Work out the finished part from the listing and answer in its coordinate system (mm). A direction names the side the tool comes from. Round coordinates to 2 decimals unless told otherwise and drop trailing zeros. Write each loop counter-clockwise with the first axis right and the second up, starting at its lowest first coordinate (ties: lowest second). Pieces come first, ordered by that corner, then holes.
from build123d import *

# Parameters (mm, degrees)
SKETCH1_W               = 160
SKETCH1_H               = 45
BOSS_EXTRUDE1_DEPTH     = 28
SKETCH3_W               = 65
SKETCH3_H               = 25
CUT_EXTRUDE2_DEPTH      = 28
CUT_EXTRUDE3_DEPTH      = 28
SKETCH8_R               = 2
CUT_EXTRUDE4_DEPTH      = 10
CUT_EXTRUDE5_DEPTH      = 169.549695936
CUT_EXTRUDE5_DEPTH_BACK = 169.549695936
SKETCH9_W               = 16
SKETCH9_H               = 28
SKETCH10_W              = 128
SKETCH10_H              = 5.5
CUT_EXTRUDE6_DEPTH      = 154.443800787
SKETCH11_W              = 128
SKETCH11_H              = 2.75
CUT_EXTRUDE7_DEPTH      = 152.921854912
SKETCH12_W              = 128
SKETCH12_H              = 2.75
BOSS_EXTRUDE3_DEPTH     = 28
SKETCH13_R              = 2
CUT_EXTRUDE8_DEPTH      = 152.230163989
SKETCH14_W              = 128
SKETCH14_H              = 28
BOSS_EXTRUDE4_DEPTH     = 2
SKETCH16_R              = 2
CUT_EXTRUDE9_DEPTH      = 152.230163989


with BuildPart() as part:
    # Sketch1 → Boss-Extrude1 (new body)
    with BuildSketch(Plane.XY):
        with Locations((80, 22.5)):
            Rectangle(SKETCH1_W, SKETCH1_H)
    extrude(amount=BOSS_EXTRUDE1_DEPTH)

    # Sketch3 → Cut-Extrude2 (cut)
    with BuildSketch(Plane.XY.offset(28)):
        with Locations((32.5, 21.5)):
            Rectangle(SKETCH3_W, SKETCH3_H)
        with Locations((127.5, 21.5)):
            Rectangle(SKETCH3_W, SKETCH3_H)
    extrude(amount=-CUT_EXTRUDE2_DEPTH, mode=Mode.SUBTRACT)

    # Sketch6 → Cut-Extrude3 (cut)
    with BuildSketch(Plane.XZ):
        Polygon((65, 14), (65, 24), (25, 24), (25, 4), (65, 4), align=None)
        Polygon((95, 4), (95, 14), (95, 24), (135, 24), (135, 4), align=None)
    extrude(amount=-CUT_EXTRUDE3_DEPTH, mode=Mode.SUBTRACT)

    # Sketch8 → Cut-Extrude4 (cut)
    with BuildSketch(Plane(origin=(0, 0, 0), x_dir=(-1, 0, 0), z_dir=(0, -1, 0))):
        with Locations(Location((-20.5, -9, 0), (0, 0, 90))):
            Circle(SKETCH8_R)
        with Locations(Location((-20.5, -19, 0), (0, 0, 90))):
            Circle(SKETCH8_R)
        with Locations(Location((-90.5, -19, 0), (0, 0, 90))):
            Circle(SKETCH8_R)
        with Locations(Location((-90.5, -9, 0), (0, 0, 90))):
            Circle(SKETCH8_R)
        with Locations(Location((-139.5, -19, 0), (0, 0, 90))):
            Circle(SKETCH8_R)
        with Locations(Location((-139.5, -9, 0), (0, 0, 90))):
            Circle(SKETCH8_R)
        with Locations(Location((-69.5, -19, 0), (0, 0, 90))):
            Circle(SKETCH8_R)
        with Locations(Location((-69.5, -9, 0), (0, 0, 90))):
            Circle(SKETCH8_R)
    extrude(amount=-CUT_EXTRUDE4_DEPTH, mode=Mode.SUBTRACT)

    # Sketch9 → Cut-Extrude5 (cut, two sides: drawn at the far end of the back side and taken through both)
    with BuildSketch(Plane(origin=(0, 0, 0), x_dir=(-1, 0, 0), z_dir=(0, -1, 0)).offset(-CUT_EXTRUDE5_DEPTH_BACK)):
        with Locations((-152, -14)):
            Rectangle(SKETCH9_W, SKETCH9_H)
        with Locations((-8, -14)):
            Rectangle(SKETCH9_W, SKETCH9_H)
    extrude(amount=CUT_EXTRUDE5_DEPTH + CUT_EXTRUDE5_DEPTH_BACK, mode=Mode.SUBTRACT)

    # Sketch10 → Cut-Extrude6 (cut, through all)
    with BuildSketch(Plane.XY.offset(28)):
        with Locations((80, 42.25)):
            Rectangle(SKETCH10_W, SKETCH10_H)
    extrude(amount=-CUT_EXTRUDE6_DEPTH, mode=Mode.SUBTRACT)

    # Sketch11 → Cut-Extrude7 (cut, through all)
    with BuildSketch(Plane.XY.offset(28)):
        with Locations((80, 38.125)):
            Rectangle(SKETCH11_W, SKETCH11_H)
    extrude(amount=-CUT_EXTRUDE7_DEPTH, mode=Mode.SUBTRACT)

    # Sketch12 → Boss-Extrude3 (add)
    with BuildSketch(Plane.XY.offset(28)):
        with Locations((80, 32.625)):
            Rectangle(SKETCH12_W, SKETCH12_H)
    extrude(amount=-BOSS_EXTRUDE3_DEPTH)

    # Sketch13 → Cut-Extrude8 (cut, through all)
    with BuildSketch(Plane(origin=(0, 36.75, 0), x_dir=(1, 0, 0), z_dir=(0, 1, 0))):
        with Locations(Location((125, -14, 0), (0, 0, 270))):
            Circle(SKETCH13_R)
        with Locations(Location((35, -14, 0), (0, 0, 270))):
            Circle(SKETCH13_R)
    extrude(amount=-CUT_EXTRUDE8_DEPTH, mode=Mode.SUBTRACT)

    # Sketch14 → Boss-Extrude4 (add)
    with BuildSketch(Plane(origin=(0, 36.75, 0), x_dir=(1, 0, 0), z_dir=(0, 1, 0))):
        with Locations((80, -14)):
            Rectangle(SKETCH14_W, SKETCH14_H)
    extrude(amount=BOSS_EXTRUDE4_DEPTH)

    # Sketch16 → Cut-Extrude9 (cut, through all)
    with BuildSketch(Plane.XZ.offset(-36.75)):
        with Locations(Location((125, 14, 0), (0, 0, 90))):
            Circle(SKETCH16_R)
        with Locations(Location((35, 14, 0), (0, 0, 90))):
            Circle(SKETCH16_R)
    extrude(amount=-CUT_EXTRUDE9_DEPTH, mode=Mode.SUBTRACT)


solid = part.part
Q1. Find section D-D (x = 90.5). Determine the outline of the cut face in (y, z), plus the area to 4 significant figures.
Q2. The mould has two halves that part along X. Classify faces 4 (the face through (144, 5, 14)), 5 (the face through (135.5, 9, 14.2)), 6 (the face through (95, 15, 14)): +X half, -X half, draft (parallel to the pull), parting line (faces both ways), or undercut.
Q3. Given pin 1 (6 mm diameter, centred on y = 13, z = 20, fed in from +X); pin 2 (12 mm diameter, centred on x = 38, y = 15.5, fed in from +Z); pin 3 (5 mm diameter, centred on x = 69.5, z = 19, fed in from -Y); pin 4 (4 mm diameter, centred on y = 20.5, z = 10.5, fed in from -X), each flat-ended and moving along its own axis, determine where each tip first touches the part or whether it passes through.
Q4. Find section B-B (z = 14). Determine the outline of the cut face in (x, y).
Q5. Find the intervals of material crossed by L1, parallel to X at y = 4, z = 21.5; L2, parallel to X at y = 26.5, z = 4.25; L3, parallel to Y at x = 119, z = 23.5, in increasing order.
Q6. A tool of negligible diameter and unlimited length cuts with its end or side. For faces 1 (the face through (79, 0, 14)), 2 (the face through (137.726, 4.437, 18.077)), 3 (the face through (65, 15, 14)), from which of +Z, -Z, +X, -X, +Y, -Y can it reach the whole face along a straight path? Write none if from no direction.
Q7. Find section A-A (x = 120.5). Determine the outline of the cut face in (y, z).
Q8. Find section C-C (x = 139.5). Determine the outline of the cut face in (y, z).
Report:
1. outline: (0, 0) - (38.75, 0) - (38.75, 28) - (0, 28) - (0, 21) - (10, 21) - (10, 17) - (0, 17) - (0, 11) - (10, 11) - (10, 7) - (0, 7) - close
1. area: 1,005 mm2
2. face 4: +X half
2. face 5: draft
2. face 6: undercut
3. pin 1: stops at x = 95
3. pin 2: passes through
3. pin 3: stops at y = 0
3. pin 4: stops at x = 65
4. outline: (16, 0) - (25, 0) - (25, 9) - (16, 9) - close; (16, 31.25) - (33, 31.25) - (33, 38.75) - (16, 38.75) - close; (37, 31.25) - (65, 31.25) - (65, 0) - (95, 0) - (95, 31.25) - (123, 31.25) - (123, 38.75) - (37, 38.75) - close; (127, 31.25) - (144, 31.25) - (144, 38.75) - (127, 38.75) - close; (135, 0) - (144, 0) - (144, 9) - (135, 9) - close
5. L1: x = 16 to 25, 65 to 95, 135 to 144
5. L2: x = 65 to 95
5. L3: y = 31.25 to 38.75
6. face 1: +Z, -Z, +X, -X, -Y
6. face 2: -Y
6. face 3: none
7. outline: (0, 0) - (9, 0) - (9, 4) - (0, 4) - close; (0, 24) - (9, 24) - (9, 28) - (0, 28) - close; (31.25, 0) - (38.75, 0) - (38.75, 28) - (31.25, 28) - close
8. outline: (0, 0) - (9, 0) - (9, 7) - (0, 7) - close; (0, 11) - (9, 11) - (9, 17) - (0, 17) - close; (0, 21) - (9, 21) - (9, 28) - (0, 28) - close; (31.25, 0) - (38.75, 0) - (38.75, 28) - (31.25, 28) - close
